Verification items for the finished model (mm, model axes). A direction names the side the tool comes from. Give positions to 0.01 mm unless a question says otherwise; leave off trailing zeros. Write each loop counter-clockwise with the first axis right and the second up, starting at its lowest first coordinate (ties: lowest second). Pieces come first, ordered by that corner, then holes.
from build123d import *

# Parameters (mm, degrees)
CROQUIS1_W              = 600
CROQUIS1_H              = 700
SALIENTE_EXTRUIR1_DEPTH = 500
CROQUIS2_R              = 12.7
SALIENTE_EXTRUIR2_DEPTH = 10
CROQUIS3_R              = 12.7


with BuildPart() as part:
    # Croquis1 → Saliente-Extruir1 (new body)
    with BuildSketch(Plane.XY):
        with Locations((300, 350)):
            Rectangle(CROQUIS1_W, CROQUIS1_H)
    extrude(amount=SALIENTE_EXTRUIR1_DEPTH)

    # Croquis2 → Saliente-Extruir2 (add)
    with BuildSketch(Plane.ZY):
        with Locations(Location((40, 30, 0), (0, 0, 180))):
            Circle(CROQUIS2_R)
    extrude(amount=SALIENTE_EXTRUIR2_DEPTH)

    # Barrer1: sweep along a curve in space
    with BuildLine() as barrer1_path:
        Line((-10, 30, 40), (-40, 30, 40))
        ThreePointArc((-40, 30, 40), (-54.142135624, 30, 34.142135624), (-60, 30, 20))
        Line((-60, 30, 20), (-60, 30, -660))
    # Croquis3 → Barrer1 (sweep)
    with BuildSketch(Plane.ZY.offset(10)):
        with Locations((40, 30)):
            Circle(CROQUIS3_R)
    sweep(path=barrer1_path.line)


solid = part.part
Item 1: Sectioned sample at C-C on z = -578. Record the cut outline in (x, y).
Answer key:
outline: circle Ø25.4 at (-60, 30)
Item 2: Sectioned sample at A-A on y = 30. Record the cut outline in (x, z).
Answer key:
outline: (-72.7, -660) - (-47.3, -660) - (-47.3, 20) arc R7.3 cw to (-40, 27.3) - (0, 27.3) - (0, 0) - (600, 0) - (600, 500) - (0, 500) - (0, 52.7) - (-40, 52.7) arc R32.7 ccw to (-72.7, 20) - close
Item 3: Sectioned sample at B-B on x = 20.5. Record the cut outline in (y, z), then the cut area to 3 significant figures.
Answer key:
outline: (0, 0) - (700, 0) - (700, 500) - (0, 500) - close
area: 350,000 mm2
Item 4: Scan lines: line 1 along Z through (x, y) = (152, 389.5); line 2 along X through (y, z) = (75.5, 53.5). Record each from-to range of solid material in increasing order.
Answer key:
line 1: z = 0 to 500
line 2: x = 0 to 600
Item 5: Release check for a two-part mould opening along X. For faces 3 (the face through (600, 345, 246)), 4 (the face through (-60, 30, -660)), 5 (the face through (-20.28, 42.672, 40.837)) record: released by +X, released by -X, zero draft, split by the parting line, or undercut.
Answer key:
face 3: released by +X
face 4: zero draft
face 5: undercut
Item 6: Set-up check for faces 1 (the face through (296, 0, 246)), 2 (the face through (-71.732, 25.136, -324.76)): record each of +Z, -Z, +X, -X, +Y, -Y from which the full face is reachable in a straight line by a thin tool's end or side.
Answer key:
face 1: +Z, -Z, +X, -X, -Y
face 2: -Z
Item 7: Depth check by flat-ended pin: pin 1 (4 mm diameter, centred on y = 480, z = 6, fed in from -X); pin 2 (10 mm diameter, centred on x = 200, z = 83, fed in from -Y); pin 3 (5 mm diameter, centred on x = 452.5, y = 246, fed in from -Z). Enter the tip coordinate at first touch or a pass-through.
Answer key:
pin 1: stops at x = 0
pin 2: stops at y = 0
pin 3: stops at z = 0
Item 8: Sectioned sample at D-D on y = 108.5. Record the cut outline in (x, z), then the cut area to 3 significant figures.
Answer key:
outline: (0, 0) - (600, 0) - (600, 500) - (0, 500) - close
area: 300,000 mm2
